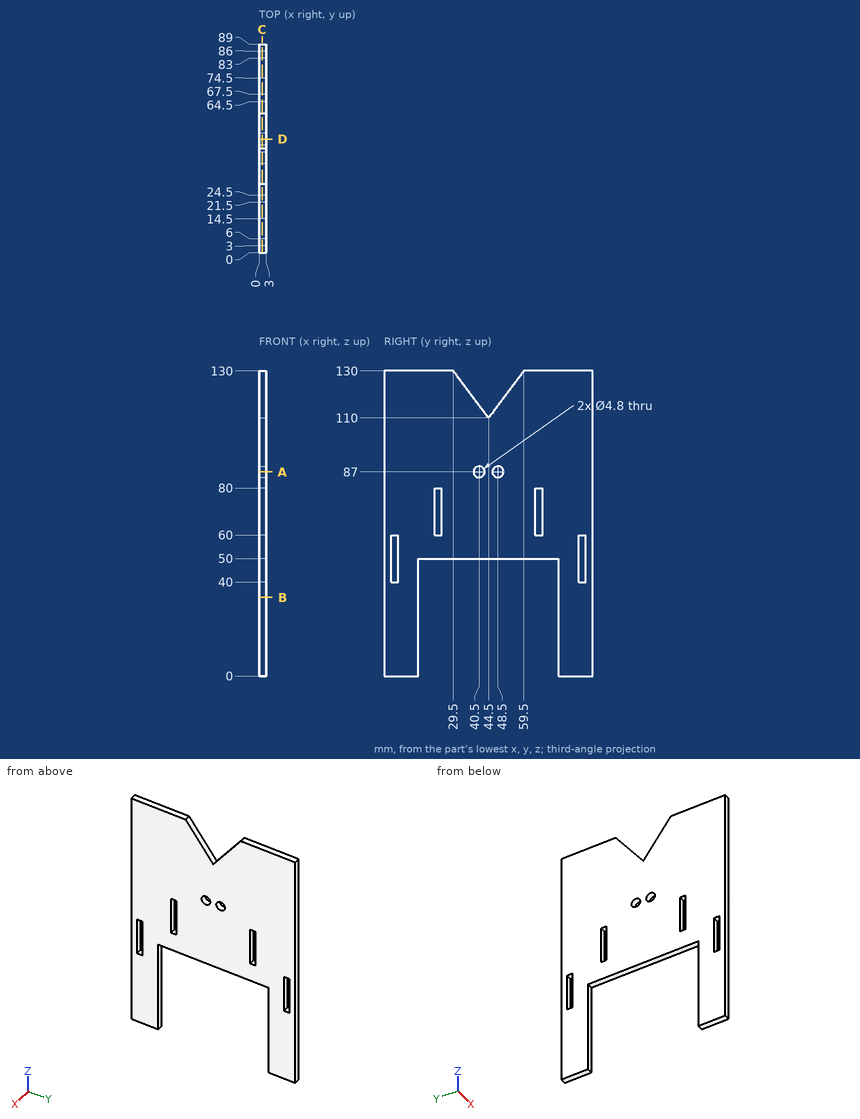
Verification items for this drawing (mm, ordinates from the low corner). Coordinates: 2 decimals unless noted, no trailing zeros. Write each loop counter-clockwise with the first axis right and the second up, starting at its lowest first coordinate (ties: lowest second). Pieces come first, ordered by that corner, then holes. Notation, with made-up numbers: (58, 60) -> (76, 60) arc R17 cw to (76, 84) -> close; hole circle Ø11 at (55, 56.25). An arc over 180 degrees is marked (long way). Use CSV: the item, a comma, the result in double quotes. Start each with the question number.
Item 1: Cross-section at D-D, the plane y = 48.5. Record the cut outline in (x, z), plus the area to 3 significant figures.
Item 2: Cross-section at A-A, the plane z = 87. Record the cut outline in (x, y).
Item 3: Thickness scan on line 1 (Y direction, x = 1.25, z = 32); line 2 (Z direction, x = 2.35, y = 67); line 3 (Z direction, x = 0.8, y = 39.5). Record the ranges inside material, lowest first.
Item 4: Cross-section at B-B, the plane z = 33.5. Record the cut outline in (x, y).
Item 5: Depth check by flat-ended pin: pin 1 Ø1.5 at (x, y) = (1, 65.5) entering from -Z; pin 2 Ø4 at (y, z) = (48.5, 87) entering from -X. Enter the tip coordinate at first touch or a pass-through.
Item 6: Cross-section at C-C, the plane x = 1.3. State how many separate pieces and enclosed holes the cut face has, plus the area to 3 significant figures.
Answers:
1,outline,"(0, 50) -> (3, 50) -> (3, 84.6) -> (0, 84.6) -> close; (0, 89.4) -> (3, 89.4) -> (3, 115.33) -> (0, 115.33) -> close"
1,area,"182 mm^2"
2,outline,"(0, 0) -> (3, 0) -> (3, 38.1) -> (0, 38.1) -> close; (0, 42.9) -> (3, 42.9) -> (3, 46.1) -> (0, 46.1) -> close; (0, 50.9) -> (3, 50.9) -> (3, 89) -> (0, 89) -> close"
3,line 1,"0 to 14.5, 74.5 to 89"
3,line 2,"50 to 60, 80 to 130"
3,line 3,"50 to 84.82, 89.18 to 116.67"
4,outline,"(0, 0) -> (3, 0) -> (3, 14.5) -> (0, 14.5) -> close; (0, 74.5) -> (3, 74.5) -> (3, 89) -> (0, 89) -> close"
5,pin 1,"z = 50"
5,pin 2,"through"
6,separate pieces,"1"
6,enclosed holes,"6"
6,area,"7,990 mm^2"
